Geometry: final body of the model. Coordinates: model frame, mm. Coordinates: 2 decimals unless noted, no trailing zeros. Write each loop counter-clockwise with the first axis right and the second up, starting at its lowest first coordinate (ties: lowest second). Pieces come first, ordered by that corner, then holes. Notation, with made-up numbers: (28.5, -27) -> (49.5, -27) arc R25 ccw to (49.5, -7) -> close; hole circle Ø1 at (-33.5, -17.5). An arc over 180 degrees is marked (long way). Answer as a JSON object with one key per item and string values. Group by question number.
```python
from build123d import *

# Parameters (mm, degrees)
SKETCH1_W      = 800
SKETCH1_H      = 600
SKETCH1_W_2    = 297
SKETCH1_H_2    = 210
EXTRUDE1_DEPTH = 10
EXTRUDE2_DEPTH = 3
SKETCH3_W      = 297
SKETCH3_H      = 5
EXTRUDE3_DEPTH = 3


with BuildPart() as part:
    # Sketch1 → Extrude1 (new body)
    with BuildSketch(Plane(origin=(0, 0, 0), x_dir=(1, 0, 0), z_dir=(0, 1, 0))):
        Rectangle(SKETCH1_W, SKETCH1_H)
        Rectangle(SKETCH1_W_2, SKETCH1_H_2, mode=Mode.SUBTRACT)
    extrude(amount=-EXTRUDE1_DEPTH)

    # Sketch2 → Extrude2 (cut)
    with BuildSketch(Plane.XZ.offset(10)):
        with BuildLine():
            Line((-148.5, -115), (-148.5, 115))
            ThreePointArc((-148.5, 115), (-151, 117.5), (-153.5, 115))
            Line((-153.5, 115), (-153.5, -115))
            ThreePointArc((-153.5, -115), (-151, -117.5), (-148.5, -115))
        make_face()
    extrude2 = extrude(amount=-EXTRUDE2_DEPTH, mode=Mode.SUBTRACT)

    # Mirror1: Extrude2 across plane
    add(extrude2.mirror(Plane(origin=(0, 0, 0), x_dir=(0, 0, 1), z_dir=(1, 0, 0))), mode=Mode.SUBTRACT)

    # Sketch3 → Extrude3 (cut)
    with BuildSketch(Plane.XZ.offset(10)):
        with Locations((0, 107.5)):
            Rectangle(SKETCH3_W, SKETCH3_H)
    extrude3 = extrude(amount=-EXTRUDE3_DEPTH, mode=Mode.SUBTRACT)

    # Mirror2: Extrude3 across plane
    add(extrude3.mirror(Plane.XY), mode=Mode.SUBTRACT)


solid = part.part
```
Item 1: Section A-A on x = 110. Output: boundary loops of the cut face in (y, z).
Item 2: Ray query, L1, parallel to Z at x = -62, y = -3; L2, parallel to X at y = -4.5, z = 37.5; L3, parallel to X at y = -7.25, z = 97.5. Return the intervals inside material, ascending. Write a range as [from, to].
Item 3: Section C-C on y = -5.5. Output: boundary loops of the cut face in (x, z).
Item 4: Section B-B on z = 44. Output: boundary loops of the cut face in (x, y).
Item 5: Mould query, pull axis Z, two halves, no side actions, for faces 1 (the flat face through (-6, 0, 129)), 2 (the flat face through (-149, -7, 1)). Classes: +Z half, -Z half, draft (parallel to the pull), parting line (faces both ways), or undercut.
Answer sheet:
{
 "1": {"outline": "(-10, -300) -> (0, -300) -> (0, -105) -> (-7, -105) -> (-7, -110) -> (-10, -110) -> close; (-10, 110) -> (-7, 110) -> (-7, 105) -> (0, 105) -> (0, 300) -> (-10, 300) -> close"},
 "2": {"L1": "z = [-300, -105], [105, 300]", "L2": "x = [-400, -148.5], [148.5, 400]", "L3": "x = [-400, -153.5], [153.5, 400]"},
 "3": {"outline": "(-400, -300) -> (400, -300) -> (400, 300) -> (-400, 300) -> close; hole (-148.5, -105) -> (148.5, -105) -> (148.5, 105) -> (-148.5, 105) -> close"},
 "4": {"outline": "(-400, -10) -> (-153.5, -10) -> (-153.5, -7) -> (-148.5, -7) -> (-148.5, 0) -> (-400, 0) -> close; (148.5, -7) -> (153.5, -7) -> (153.5, -10) -> (400, -10) -> (400, 0) -> (148.5, 0) -> close"},
 "5": {"face 1": "draft", "face 2": "undercut"}
}
